from build123d import *

# Parameters (mm, degrees)
SKETCH1_W                  = 340
SKETCH1_H                  = 550
BOSS_EXTRUDE1_DEPTH        = 1.3
F_20_0_20_DIAMETER_HOLE1_D = 20
F_5_0_5_DIAMETER_HOLE1_D   = 5
CONVERT_SOLID1_START       = -0.2
CONVERT_SOLID1_OUTLINE_W   = 340
CONVERT_SOLID1_OUTLINE_H   = 550
CONVERT_SOLID1_OUTLINE_R   = 2.5
CONVERT_SOLID1_OUTLINE_R_2 = 10
CONVERT_SOLID1_DEPTH       = 0.2
SKETCHED_START             = -275
SKETCHED_BEND1_OUTLINE_W   = 1.5
SKETCHED_BEND1_OUTLINE_H   = 340
SKETCHED_BEND1_DEPTH       = 50.30822
SKETCHED_START_2           = -225
SKETCHED_BEND1_2_OUTLINE_W = 50.965708265
SKETCHED_BEND1_2_OUTLINE_H = 340
SKETCHED_BEND1_2_OUTLINE_R = 2.5
SKETCHED_BEND1_2_DEPTH     = 3
SKETCHED_START_3           = -171
SKETCHED_BEND1_3_DEPTH     = 342
CUT_EXTRUDE1_DEPTH         = 328.32694619
CUT_EXTRUDE1_DEPTH_BACK    = 328.32694619
SKETCH1_3_R                = 1.5


with BuildPart() as part:
    # Sketch1 → Boss-Extrude1 (new body)
    with BuildSketch(Plane.YZ):
        Rectangle(SKETCH1_W, SKETCH1_H)
    extrude(amount=BOSS_EXTRUDE1_DEPTH)

    # Ø20.0 (20) Diameter Hole1 (through all)
    with Locations(Plane.YZ.offset(1.3)):
        with Locations((80, -25), (40, -25), (120, -25), (0, -25), (-40, -25), (-80, -25), (120, 75), (80, 75), (40, 75), (0, 75), (-40, 75), (-80, 75), (120, 175), (80, 175), (40, 175), (0, 175), (-40, 175), (-80, 175)):
            Hole(F_20_0_20_DIAMETER_HOLE1_D / 2)

    # Ø5.0 (5) Diameter Hole1 (through all)
    with Locations(Plane.YZ.offset(1.3)):
        with Locations((157.3, -139.45), (20, -139.45), (-117.3, -139.45), (140, -250), (0, -250), (-140, -250)):
            Hole(F_5_0_5_DIAMETER_HOLE1_D / 2)

    # Convert-Solid1: read off the stored shape, not the designer's step
    # Convert-Solid1 outline → Convert-Solid1 (add)
    with BuildSketch(Plane.YZ.offset(CONVERT_SOLID1_START)):
        Rectangle(CONVERT_SOLID1_OUTLINE_W, CONVERT_SOLID1_OUTLINE_H)
        with Locations((-140, -250)):
            Circle(CONVERT_SOLID1_OUTLINE_R, mode=Mode.SUBTRACT)
        with Locations((-117.3, -139.45)):
            Circle(CONVERT_SOLID1_OUTLINE_R, mode=Mode.SUBTRACT)
        with Locations((-80, -25)):
            Circle(CONVERT_SOLID1_OUTLINE_R_2, mode=Mode.SUBTRACT)
        with Locations((-40, -25)):
            Circle(CONVERT_SOLID1_OUTLINE_R_2, mode=Mode.SUBTRACT)
        with Locations((0, -250)):
            Circle(CONVERT_SOLID1_OUTLINE_R, mode=Mode.SUBTRACT)
        with Locations((20, -139.45)):
            Circle(CONVERT_SOLID1_OUTLINE_R, mode=Mode.SUBTRACT)
        with Locations((140, -250)):
            Circle(CONVERT_SOLID1_OUTLINE_R, mode=Mode.SUBTRACT)
        with Locations((157.3, -139.45)):
            Circle(CONVERT_SOLID1_OUTLINE_R, mode=Mode.SUBTRACT)
        with Locations((0, -25)):
            Circle(CONVERT_SOLID1_OUTLINE_R_2, mode=Mode.SUBTRACT)
        with Locations((40, -25)):
            Circle(CONVERT_SOLID1_OUTLINE_R_2, mode=Mode.SUBTRACT)
        with Locations((80, -25)):
            Circle(CONVERT_SOLID1_OUTLINE_R_2, mode=Mode.SUBTRACT)
        with Locations((120, -25)):
            Circle(CONVERT_SOLID1_OUTLINE_R_2, mode=Mode.SUBTRACT)
        with Locations((-80, 75)):
            Circle(CONVERT_SOLID1_OUTLINE_R_2, mode=Mode.SUBTRACT)
        with Locations((-40, 75)):
            Circle(CONVERT_SOLID1_OUTLINE_R_2, mode=Mode.SUBTRACT)
        with Locations((-80, 175)):
            Circle(CONVERT_SOLID1_OUTLINE_R_2, mode=Mode.SUBTRACT)
        with Locations((-40, 175)):
            Circle(CONVERT_SOLID1_OUTLINE_R_2, mode=Mode.SUBTRACT)
        with Locations((0, 75)):
            Circle(CONVERT_SOLID1_OUTLINE_R_2, mode=Mode.SUBTRACT)
        with Locations((40, 75)):
            Circle(CONVERT_SOLID1_OUTLINE_R_2, mode=Mode.SUBTRACT)
        with Locations((80, 75)):
            Circle(CONVERT_SOLID1_OUTLINE_R_2, mode=Mode.SUBTRACT)
        with Locations((120, 75)):
            Circle(CONVERT_SOLID1_OUTLINE_R_2, mode=Mode.SUBTRACT)
        with Locations((0, 175)):
            Circle(CONVERT_SOLID1_OUTLINE_R_2, mode=Mode.SUBTRACT)
        with Locations((40, 175)):
            Circle(CONVERT_SOLID1_OUTLINE_R_2, mode=Mode.SUBTRACT)
        with Locations((80, 175)):
            Circle(CONVERT_SOLID1_OUTLINE_R_2, mode=Mode.SUBTRACT)
        with Locations((120, 175)):
            Circle(CONVERT_SOLID1_OUTLINE_R_2, mode=Mode.SUBTRACT)
    extrude(amount=CONVERT_SOLID1_DEPTH)

    # Sketched Bend1: read off the stored shape, not the designer's step
    # Sketched Bend1 outline → Sketched Bend1 (cut)
    with BuildSketch(Plane.XY.offset(SKETCHED_START)):
        with Locations((0.55, 0)):
            Rectangle(SKETCHED_BEND1_OUTLINE_W, SKETCHED_BEND1_OUTLINE_H)
    extrude(amount=SKETCHED_BEND1_DEPTH, mode=Mode.SUBTRACT)

    # Sketched Bend1 2 outline → Sketched Bend1 2 (add)
    with BuildSketch(Plane.XY.offset(SKETCHED_START_2)):
        with Locations((-25.682854133, 0)):
            Rectangle(SKETCHED_BEND1_2_OUTLINE_W, SKETCHED_BEND1_2_OUTLINE_H)
        with Locations((-26.165708265, -140)):
            Circle(SKETCHED_BEND1_2_OUTLINE_R, mode=Mode.SUBTRACT)
        with Locations((-26.165708265, 0)):
            Circle(SKETCHED_BEND1_2_OUTLINE_R, mode=Mode.SUBTRACT)
        with Locations((-26.165708265, 140)):
            Circle(SKETCHED_BEND1_2_OUTLINE_R, mode=Mode.SUBTRACT)
    extrude(amount=SKETCHED_BEND1_2_DEPTH)

    # Sketched Bend1 3 outline → Sketched Bend1 3 (cut)
    with BuildSketch(Plane(origin=(0, 0, 0), x_dir=(1, 0, 0), z_dir=(0, 1, 0)).offset(SKETCHED_START_3)):
        with BuildLine():
            ThreePointArc((-0.2, 222), (-0.639339828, 223.060660172), (-1.7, 223.5))
            Line((-1.7, 223.5), (-51.165708265, 223.5))
            Line((-51.165708265, 223.5), (-51.165708265, 222))
            Line((-51.165708265, 222), (-0.2, 222))
        make_face()
        with BuildLine():
            Line((-0.2, 225), (-1.7, 225))
            ThreePointArc((-1.7, 225), (0.421320344, 224.121320344), (1.3, 222))
            Line((1.3, 222), (1.3, 224.69178))
            Line((1.3, 224.69178), (-0.2, 224.69178))
            Line((-0.2, 224.69178), (-0.2, 225))
        make_face()
    extrude(amount=SKETCHED_BEND1_3_DEPTH, mode=Mode.SUBTRACT)

    # Sketch1<3> → Cut-Extrude1 (cut, two sides: drawn at the far end of the back side and taken through both)
    with BuildSketch(Plane.YZ.offset(-CUT_EXTRUDE1_DEPTH_BACK)):
        with Locations(Location((-132.789034574, 262.3, 0), (0, 0, 270))):
            Circle(SKETCH1_3_R)
        with Locations(Location((-156.891480577, 262.3, 0), (0, 0, 270))):
            Circle(SKETCH1_3_R)
    extrude(amount=CUT_EXTRUDE1_DEPTH + CUT_EXTRUDE1_DEPTH_BACK, mode=Mode.SUBTRACT)


solid = part.part
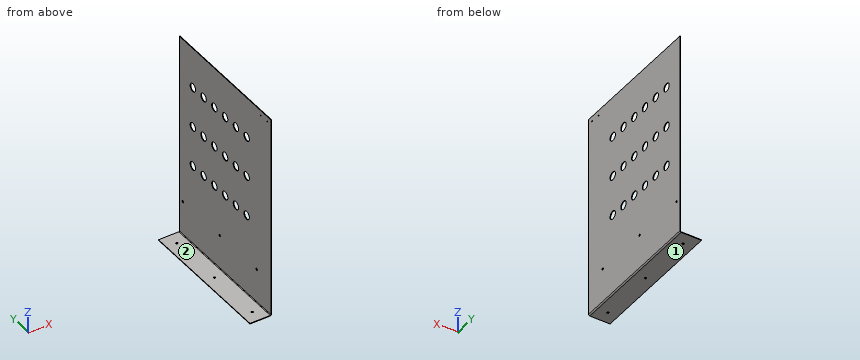
Work out the finished part from the listing and answer in its coordinate system (mm). Face numbers are marked on the shaded views. A direction names the side the tool comes from. Round coordinates to 2 decimals unless told otherwise and drop trailing zeros. Order: outer loops, then holes, each group sorted by start corner. A loop starts at its lowest first (then second) coordinate and runs counter-clockwise, first axis right, second up. Notation, with made-up numbers: M -1,75.25 L 36,75.25 A19 cw 36,83.25 Z; hole C 66.5,44.5 d3. An arc over 180 degrees is marked long. One line per item, written item: value.
Q1. Find section B-B on y = 120. Write down the section's boundary in (x, z), then the cut area to 3 significant figures.
Derived:
outline: M -51.17,-225 L -1.7,-225 A3 ccw 1.3,-222 L 1.3,-35 L -0.2,-35 L -0.2,-222 A1.5 cw -1.7,-223.5 L -51.17,-223.5 Z; M -0.2,-15 L 1.3,-15 L 1.3,65 L -0.2,65 Z; M -0.2,85 L 1.3,85 L 1.3,165 L -0.2,165 Z; M -0.2,185 L 1.3,185 L 1.3,275 L -0.2,275 Z
area: 735 mm²
Q2. Straight lines are drawn through the part: line 1 (Z direction, x = 0.4, y = 120); line 2 (X direction, y = 65, z = -65.5); line 3 (Z direction, x = 1, y = 80). For each, find the intervals that lie inside material, in ascending order.
Derived:
line 1: -224.14 to -35, -15 to 65, 85 to 165, 185 to 275
line 2: -0.2 to 1.3
line 3: -223.31 to -35, -15 to 65, 85 to 165, 185 to 275
Q3. Find section A-A on z = -25. Write down the section's boundary in (x, y).
Derived:
outline: M -0.2,-170 L 1.3,-170 L 1.3,-90 L -0.2,-90 Z; M -0.2,-70 L 1.3,-70 L 1.3,-50 L -0.2,-50 Z; M -0.2,-30 L 1.3,-30 L 1.3,-10 L -0.2,-10 Z; M -0.2,10 L 1.3,10 L 1.3,30 L -0.2,30 Z; M -0.2,50 L 1.3,50 L 1.3,70 L -0.2,70 Z; M -0.2,90 L 1.3,90 L 1.3,110 L -0.2,110 Z; M -0.2,130 L 1.3,130 L 1.3,170 L -0.2,170 Z
Q4. Find section D-D on z = 195. Write down the section's boundary in (x, y).
Derived:
outline: M -0.2,-170 L 1.3,-170 L 1.3,170 L -0.2,170 Z
Q5. Find section C-C on y = -39. Write down the section's boundary in (x, z), then the cut area to 3 significant figures.
Derived:
outline: M -51.17,-225 L -1.7,-225 A3 ccw 1.3,-222 L 1.3,-34.95 L -0.2,-34.95 L -0.2,-222 A1.5 cw -1.7,-223.5 L -51.17,-223.5 Z; M -0.2,-15.05 L 1.3,-15.05 L 1.3,65.05 L -0.2,65.05 Z; M -0.2,84.95 L 1.3,84.95 L 1.3,165.05 L -0.2,165.05 Z; M -0.2,184.95 L 1.3,184.95 L 1.3,275 L -0.2,275 Z
area: 735 mm²
Q6. Flat-ended cylindrical pins translate along their axes: pin 1 (8 mm diameter, centred on y = -30, z = -59, fed in from -X); pin 2 (8 mm diameter, centred on x = -26.17, y = -140, fed in from +Z). Find the tip coordinate at first contact, or state that the pin passes through.
Derived:
pin 1: x = -0.2
pin 2: z = -223.5
Q7. For the marked faces 1 and 2, determine the directions among +Z, -Z, +X, -X, +Y, -Y from which every point of the face is accessible in a straight line to the end or side of a thin tool.
Derived:
face 1: -Z, +X, -X, +Y, -Y
face 2: +Z, -X, +Y, -Y
